from build123d import *

# Parameters (mm, degrees)
SKETCH1_R               = 7
BOSS_EXTRUDE1_DEPTH     = 8
SKETCH2_R               = 6
BOSS_EXTRUDE2_DEPTH     = 14
SKETCH6_R               = 3
CUT_EXTRUDE2_DEPTH      = 20
CUT_EXTRUDE3_REACH      = 29
CUT_EXTRUDE3_END_RADIUS = 3
SKETCH8_R               = 1
CIRPATTERN1_COUNT       = 2
CIRPATTERN1_ANGLE       = 90
FILLET1_R               = 0.5
SKETCH3_R               = 7
CUT_EXTRUDE_2_DEPTH     = 2
SCALE_1_SCALE           = 0.894736842
SKETCH_1_R              = 3
CUT_EXTRUDE_3_DEPTH     = 20.969059417


with BuildPart() as part:
    # Sketch1 → Boss-Extrude1 (new body)
    with BuildSketch(Plane(origin=(0, 0, 0), x_dir=(1, 0, 0), z_dir=(0, 1, 0))):
        with Locations(Location((0, 0, 0), (0, 0, 270))):
            Circle(SKETCH1_R)
    extrude(amount=BOSS_EXTRUDE1_DEPTH)

    # Sketch2 → Boss-Extrude2 (add)
    with BuildSketch(Plane(origin=(0, 8, 0), x_dir=(1, 0, 0), z_dir=(0, 1, 0))):
        with Locations(Location((0, 0, 0), (0, 0, 270))):
            Circle(SKETCH2_R)
    extrude(amount=BOSS_EXTRUDE2_DEPTH)

    # Sketch6 → Cut-Extrude2 (cut)
    with BuildSketch(Plane.XZ):
        with Locations(Location((0, 0, 0), (0, 0, 270))):
            Circle(SKETCH6_R)
    extrude(amount=-CUT_EXTRUDE2_DEPTH, mode=Mode.SUBTRACT)

    # Cut-Extrude3: up to this cylinder (the profile starts outside it)
    cut_extrude3_end = Plane(origin=(0, 4, 0), z_dir=(0, -1, 0)) * Cylinder(CUT_EXTRUDE3_END_RADIUS, 65, mode=Mode.PRIVATE)
    # Sketch8 → Cut-Extrude3 (cut, up to the surface)
    with BuildSketch(Plane.XY.offset(7), mode=Mode.PRIVATE) as cut_extrude3_sk1:
        with Locations((0, 4)):
            Circle(SKETCH8_R)
    cut_extrude3_tool1 = extrude(cut_extrude3_sk1.sketch, amount=-CUT_EXTRUDE3_REACH, mode=Mode.PRIVATE) - cut_extrude3_end
    cut_extrude3 = cut_extrude3_tool1.solids().sort_by_distance((0, 4, 7))[0]
    add(cut_extrude3, mode=Mode.SUBTRACT)

    # CirPattern1: Cut-Extrude3 ×2 about axis
    cirpattern1_axis = Axis((0, 0, 0), (0, 1, 0))
    for i in range(1, CIRPATTERN1_COUNT):
        add(cut_extrude3.rotate(cirpattern1_axis, i * CIRPATTERN1_ANGLE / (CIRPATTERN1_COUNT - 1)), mode=Mode.SUBTRACT)

    # Fillet1
    fillet1_edges = [part.edges().sort_by_distance(p)[0] for p in [
        (-1, 4, 6.92820323),
        (6.92820323, 4, 1),
    ]]
    fillet(fillet1_edges, radius=FILLET1_R)

    # Sketch3 → ｶｯﾄ - 押し出し2 (cut)
    with BuildSketch(Plane(origin=(0, 22, 0), x_dir=(1, 0, 0), z_dir=(0, 1, 0))):
        with Locations(Location((0, 0, 0), (0, 0, 270))):
            Circle(SKETCH3_R)
    extrude(amount=-CUT_EXTRUDE_2_DEPTH, mode=Mode.SUBTRACT)


with BuildPart() as part_1:
    # ｽｹｰﾙ1: scaled about (-0.033116377, 9.097196925, -0.033121406)
    add(part.part.scale(SCALE_1_SCALE).moved(Location((-0.003485934, 0.957599676, -0.003486464))))

    # ｽｹｯﾁ1 → ｶｯﾄ - 押し出し3 (cut, through all)
    with BuildSketch(Plane.XZ.offset(-0.957597864)):
        with Locations(Location((0, 0, 0), (0, 0, 270))):
            Circle(SKETCH_1_R)
    extrude(amount=-CUT_EXTRUDE_3_DEPTH, mode=Mode.SUBTRACT)


solid = part_1.part
Work out the finished part from the listing and answer in its coordinate system (mm). A direction names the side the tool comes from. Coordinates: 2 decimals unless noted, no trailing zeros. Write each loop counter-clockwise with the first axis right and the second up, starting at its lowest first coordinate (ties: lowest second). Pieces come first, ordered by that corner, then holes.
1. The part is cut by section C-C, the plane z = -2.5. Write down the section's boundary in (x, y).
Results list:
outline: (-5.75, 0.96) - (-1.66, 0.96) - (-1.66, 18.85) - (-4.76, 18.85) - (-4.76, 8.12) - (-5.75, 8.12) - close; (1.66, 0.96) - (5.74, 0.96) - (5.74, 8.12) - (4.75, 8.12) - (4.75, 18.85) - (1.66, 18.85) - close
2. Flat-ended cylindrical pins translate along their axes: pin 1 (1 mm diameter, centred on x = 4, y = 4.5, fed in from -Z); pin 2 (3 mm diameter, centred on x = -2.5, y = 16, fed in from -Z); pin 3 (2 mm diameter, centred on y = 4, z = 1.5, fed in from +X). Find the tip coordinate at first contact, or state that the pin passes through.
Results list:
pin 1: stops at z = -5.2
pin 2: stops at z = -5.28
pin 3: stops at x = 6.22
3. The part is cut by section B-B, the plane z = 0. State how many separate pieces and enclosed holes the cut face has, and give its area (3 significant figures).
Results list:
separate pieces: 3
enclosed holes: 0
area: 91.7 mm2
4. For faces 4 (the cylindrical face through (4.359, 3.743, -0.416)), 5 (the flat face through (-2.3, 18.852, 2.3)), 6 (the cylindrical face through (0.82, 4.19, 4.36)), determine the directions among +Z, -Z, +X, -X, +Y, -Y from which every point of the face is accessible in a straight line to the end or side of a thin tool.
Results list:
face 4: +X
face 5: +Z, -Z, +X, -X, +Y
face 6: +Z
5. For a pull along Z with two mould halves and no side action, classify faces 1 (the cylindrical face through (-1.15, 9.78, -2.77)), 2 (the cylindrical face through (-3.27, 13.409, -4.264)), 3 (the flat face through (3, 8.115, 5)) as +Z half, -Z half, draft (parallel to the pull), parting line (faces both ways), or undercut.
Results list:
face 1: undercut
face 2: parting line
face 3: draft
6. Consider line 1 along Z through (x, y) = (0, 15.5); line 2 along Z through (x, y) = (0, 7.25); line 3 along X through (y, z) = (5.5, 0). Determine where each line is inside the solid, lowest interval first.
Results list:
line 1: z = -5.37 to -3, 3 to 5.36
line 2: z = -6.27 to -3, 3 to 6.26
line 3: x = -6.27 to -3, 3 to 6.05
7. The part is cut by section D-D, the plane y = 11.25. Write down the section's boundary in (x, z), and give its area (3 significant figures).
Results list:
outline: circle Ø10.74 at (0, 0); hole circle Ø6 at (0, 0)
area: 62.3 mm2
8. The part is cut by section A-A, the plane x = -2.25. Write down the section's boundary in (y, z).
Results list:
outline: (0.96, -5.85) - (8.12, -5.85) - (8.12, -4.88) - (18.85, -4.88) - (18.85, -1.98) - (0.96, -1.98) - close; (0.96, 1.98) - (18.85, 1.98) - (18.85, 4.87) - (8.12, 4.87) - (8.12, 5.84) - (0.96, 5.84) - close
